Answer from the drawing. Dimensions are ordinates in mm from the lowest x, y and z of the part. A direction names the side the tool comes from. Coordinates: 2 decimals unless noted, no trailing zeros. Write each loop counter-clockwise with the first axis right and the second up, starting at its lowest first coordinate (ties: lowest second). Pieces come first, ordered by that corner, then holes.
1) Each of these flat-tipped pins is pushed along its axis until it touches: pin 1 Ø1 at (x, z) = (53.5, 8.5) entering from +Y; pin 2 Ø6 at (y, z) = (19.5, 15.5) entering from +X; pin 3 Ø10 at (y, z) = (62.5, 6) entering from -X. Where does it stop, or does it pass through?
2) The part is cut by section D-D (z = 8.25). Determine the outline of the cut face in (x, y).
3) The part is cut by section A-A (x = 46.5). Determine the outline of the cut face in (y, z).
4) Find the intervals of material crossed by line 1 (Y direction, x = 46.5, z = 4); line 2 (Y direction, x = 46.5, z = 8.5); line 3 (Z direction, x = 76.5, y = 70), in increasing order.
5) Determine the mould class of the marked faces 3, 4 and 5 for opening direction Y: +Y half, -Y half, draft (parallel to the pull), parting line (faces both ways), or undercut.
6) The part is cut by section B-B (y = 66.5). Determine the outline of the cut face in (x, z).
7) Which of the six approach directions +Z, -Z, +X, -X, +Y, -Y give full straight-line access (tool end or side, diameter ignored) to the marked faces 1 and 2?
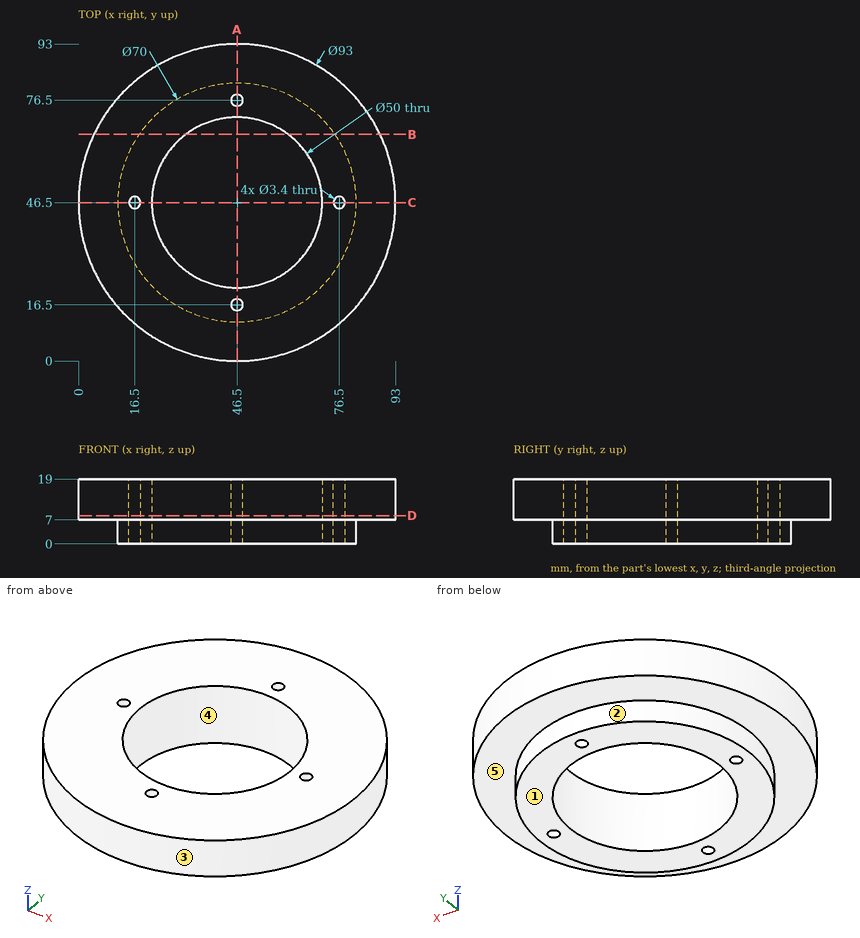
Reported:
1. pin 1: stops at y = 92.54
1. pin 2: stops at x = 86.33
1. pin 3: stops at x = 1.34
2. outline: circle Ø93 at (46.5, 46.5); hole circle Ø3.4 at (16.5, 46.5); hole circle Ø50 at (46.5, 46.5); hole circle Ø3.4 at (46.5, 16.5); hole circle Ø3.4 at (46.5, 76.5); hole circle Ø3.4 at (76.5, 46.5)
3. outline: (0, 7) - (11.5, 7) - (11.5, 0) - (14.8, 0) - (14.8, 19) - (0, 19) - close; (18.2, 0) - (21.5, 0) - (21.5, 19) - (18.2, 19) - close; (71.5, 0) - (74.8, 0) - (74.8, 19) - (71.5, 19) - close; (78.2, 0) - (81.5, 0) - (81.5, 7) - (93, 7) - (93, 19) - (78.2, 19) - close
4. line 1: y = 11.5 to 14.8, 18.2 to 21.5, 71.5 to 74.8, 78.2 to 81.5
4. line 2: y = 0 to 14.8, 18.2 to 21.5, 71.5 to 74.8, 78.2 to 93
4. line 3: z = 7 to 19
5. face 3: parting line
5. face 4: undercut
5. face 5: draft
6. outline: (4.52, 7) - (17.78, 7) - (17.78, 0) - (31.5, 0) - (31.5, 19) - (4.52, 19) - close; (61.5, 0) - (75.22, 0) - (75.22, 7) - (88.48, 7) - (88.48, 19) - (61.5, 19) - close
7. face 1: -Z, +X, -X, +Y, -Y
7. face 2: -Z
